Autodesk Inventor part; units mm, degrees
ref_plane "Work Plane1" through (-7.9612, 0, 0) normal (0, -0.866, -0.5) x (1, 0, 0)
ref_plane "YZ Plane" through (0, 0, 0) normal (1, 0, 0) x (0, 1, 0)
ref_plane "XZ Plane" through (0, 0, 0) normal (0, 1, 0) x (-1, 0, 0)
sketch "Sketch1" plane through (0, 0, 0) normal (1, 0, 0) x (0, 1, 0)
  line L0 (-4.0415, 0) -> (-2.0207, 3.5)
  line L1 (-2.0207, 3.5) -> (2.0207, 3.5)
  line L2 (2.0207, 3.5) -> (4.0415, 0)
  line L3 (4.0415, 0) -> (2.0207, -3.5)
  line L4 (2.0207, -3.5) -> (-2.0207, -3.5)
  line L5 (-2.0207, -3.5) -> (-4.0415, 0)
  point P0 (0, 0)
  point P1 (0, 0)
  dimension "d0" = 8.0829
extrude "Body" add sketch "Sketch1" along normal blind 3.2
sketch "Sketch2" plane through (0, 0, 0) normal (0, 0, 1) x (1, 0, 0)
  line L0 (0, 2.0207) -> (0, 4.0415)
  line L1 (0, 4.0415) -> (3.2, 4.0415)
  line L2 (3.2, 2.0207) -> (3.2, 4.0415)
  line L3 (-0.64, 0) -> (3.84, 0)
  line L4 (0.6302, 4.0415) -> (0, 2.95)
  line L5 (2.5698, 4.0415) -> (3.2, 2.95)
  dimension "d3" = 30
  dimension "d4" = 30
  dimension "d5" = 5.9
  dimension "d6" = 5.9
revolve "Chamfer1" cut sketch "Sketch2" angle 360 about axis through (-10, 0, 0) along (1, 0, 0)
sketch "Sketch3" plane through (3.2, 0, 0) normal (1, 0, 0) x (0, 0, -1)
  arc A0 (-0.625, -1.0825) -> (0.625, -1.0825) centre (0, 0) ccw
hole "Thread" at (3.2, 0, 0) direction (-1, 0, 0) diameter 3.242 end through all
chamfer "Chamfer2" distance 0.3789 angle 30 1 edges at (3.2, 0, 1.621) measured on face at (3.2, 2.4745, -0.3005)
chamfer "Chamfer3" distance 0.3789 angle 30 1 edges at (0, 0, 1.621) measured on face at (0, 2.4745, -0.3005)
ref_plane "Work Plane1" through (-7.9612, 0, 0) normal (0, -0.866, -0.5) x (1, 0, 0)
equation "\"d0\" = 1.1547 * SW"
equation "\"d1\" = KOH"
equation "\"d3\" = ANG1"
equation "\"d4\" = ANG2"
equation "\"d5\" = SW0"
equation "\"d6\" = SW01"
equation "\"d8\" = -0.5 * GD1 + 0.5 * NND"
equation "\"d40\" = -0.5 * GD1 + 0.5 * NND"
equation "\"d10\" = -0.5 * GD1 + 0.5 * NND"
equation "\"d41\" = -0.5 * GD1 + 0.5 * NND"
equation "\"ANG1\" = 30deg"
equation "\"ANG2\" = 30deg"
equation "\"NND\" = 4"
equation "\"KOH\" = 3.2"
equation "\"SW\" = 7"
equation "\"SW0\" = 5.9"
equation "\"SW01\" = 5.9"
equation "\"GUL\" = 0.541266 * PTC"
equation "\"THREADDIA\" = 4"
equation "\"TOA\" = 30deg"
equation "\"PTC\" = 0.7"
equation "\"E0\" = 1.155 * SW"
equation "\"GAL\" = 0.541266 * PTC"
properties part number "ISO 4032 - M4" material "Stainless Steel, 440C"
Model file for the job. Use its own axes, mm. Coordinates: 2 decimals unless noted, no trailing zeros. Write each loop counter-clockwise with the first axis right and the second up, starting at its lowest first coordinate (ties: lowest second). Pieces come first, ordered by that corner, then holes. Notation, with made-up numbers: (32, -15) -> (80, -15) arc R24 cw to (80, 3) -> close; hole circle Ø11 at (44.25, 24.5). An arc over 180 degrees is marked (long way). One line per item, written item: value. Start each with the question number.
1) Probe probe 1 along Z at (x, y) = (1.2, 0); probe 2 along Z at (x, y) = (2.6, 0.5); probe 3 along Y at (x, z) = (0.35, 0.75). List the from-to ranges inside material, lowest first.
2) Slice it at A-A on y = 0. Write the cut outline in (x, z).
3) Slice it at B-B on x = 1.45. Write the cut outline in (y, z).
4) Pull direction Z, two halves, no side cores. Call faces 1 (the face through (1.6, -3, -1.8)), 2 (the face through (3.2, 2, -1)), 3 (the face through (1.581, 1.438, -0.748)), 4 (the face through (1.6, 3, 1.8)): +Z half, -Z half, draft (parallel to the pull), parting line (faces both ways), or undercut.
5) Slice it at C-C on x = 0.45. Write the cut outline in (y, z).
6) Flat gauge pins, fed straight in: pin 1 Ø2.5 at (y, z) = (0, 0) entering from +X; pin 2 Ø1 at (x, z) = (0.5, -1) entering from +Y; pin 3 Ø1 at (x, z) = (1, 2) entering from +Y. Where does each tip first touch, or does it go through?
Answers follow:
1. probe 1: -3.5 to -1.62, 1.62 to 3.5
1. probe 2: -3.5 to -1.54, 1.54 to 3.5
1. probe 3: -3.48 to -1.44, 1.44 to 3.48
2. outline: (0, -2.95) -> (0.32, -3.5) -> (2.88, -3.5) -> (3.2, -2.95) -> (3.2, -2) -> (2.98, -1.62) -> (0.22, -1.62) -> (0, -2) -> close; (0, 2) -> (0.22, 1.62) -> (2.98, 1.62) -> (3.2, 2) -> (3.2, 2.95) -> (2.88, 3.5) -> (0.32, 3.5) -> (0, 2.95) -> close
3. outline: (-4.04, 0) -> (-2.02, -3.5) -> (2.02, -3.5) -> (4.04, 0) -> (2.02, 3.5) -> (-2.02, 3.5) -> close; hole circle Ø3.24 at (0, 0)
4. face 1: -Z half
4. face 2: draft
4. face 3: undercut
4. face 4: +Z half
5. outline: (-3.67, -0.63) -> (-2.39, -2.87) arc R3.73 ccw to (-1.29, -3.5) -> (1.29, -3.5) arc R3.73 ccw to (2.39, -2.87) -> (3.67, -0.63) arc R3.73 ccw to (3.67, 0.63) -> (2.39, 2.87) arc R3.73 ccw to (1.29, 3.5) -> (-1.29, 3.5) arc R3.73 ccw to (-2.39, 2.87) -> (-3.67, 0.63) arc R3.73 ccw to start; hole circle Ø3.24 at (0, 0)
6. pin 1: through
6. pin 2: y = 3.75
6. pin 3: y = 3.18
